Geometry check sheet. Reference: drawing and pictorial views, mm from the part's lowest x, y, z. A direction names the side the tool comes from. Round coordinates to 2 decimals unless told otherwise and drop trailing zeros. Loops run counter-clockwise (first coordinate to the right, second up) from the corner with the lowest first, then second, coordinate; pieces in that order, holes last. Notation, with made-up numbers: (-12.75, 76) -> (11.25, 76) arc R20 cw to (11.25, 87) -> close; hole circle Ø5 at (-23, -10.75). An arc over 180 degrees is marked (long way). Use one line per item in the form item = value. Start each with the question number.
(1) Material ranges on probe 1 along Z at (x, y) = (5.5, 6.5); probe 2 along Y at (x, z) = (3, 18.75); probe 3 along Y at (x, z) = (17, 18.75), recorded low to high. Write a range as [from, to].
(2) Draft check along X on the marked faces 1, 2 and 3. Enter one of: released by +X, released by -X, zero draft, split by the parting line, or undercut.
(3) Sectioned sample at B-B (x = 3). Record the cut outline in (y, z).
(4) Sectioned sample at D-D (x = 10). Record the cut outline in (y, z), and give its area (3 significant figures).
(5) Sectioned sample at C-C (z = 15.5). Record the cut outline in (x, y), and give its area (3 significant figures).
(6) Set-up check for the marked faces 4, 5 and 6: record each of +Z, -Z, +X, -X, +Y, -Y from which the full face is reachable in a straight line by a thin tool's end or side.
(7) Go/stop test with flat-tipped pins: pin 1 (1 mm diameter, centred on x = 10.5, z = 11, fed in from -Y); pin 2 (5 mm diameter, centred on y = 21, z = 6, fed in from +X) (3 decimals); pin 3 (1 mm diameter, centred on x = 9.5, y = 15, fed in from +Z). Record where each tip stops, or that it passes through.
(8) Sectioned sample at A-A (z = 24.25). Record the cut outline in (x, y).
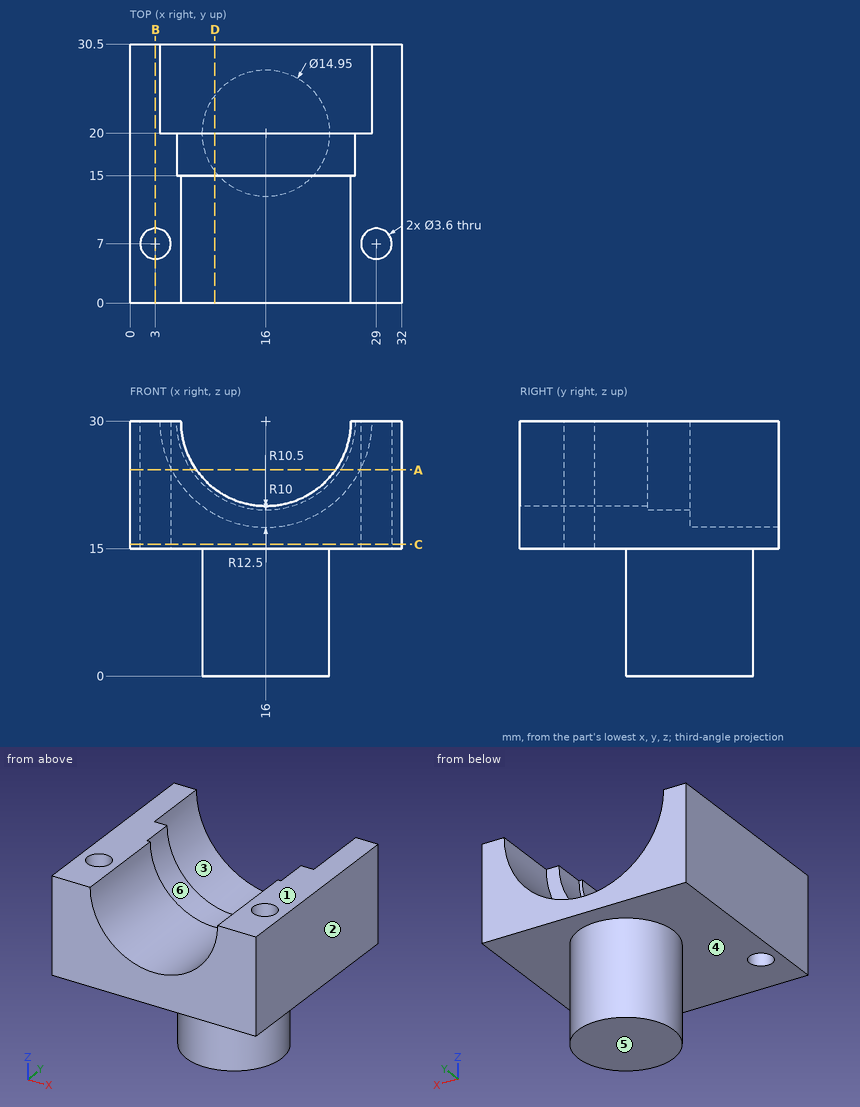
Checks:
q1.probe_1 = [15, 30]
q1.probe_2 = [0, 5.2], [8.8, 30.5]
q1.probe_3 = [0, 20]
q2.face_1 = zero draft
q2.face_2 = released by +X
q2.face_3 = undercut
q3.outline = (0, 15) -> (5.2, 15) -> (5.2, 30) -> (0, 30) -> close; (8.8, 15) -> (30.5, 15) -> (30.5, 30) -> (8.8, 30) -> close
q4.outline = (0, 15) -> (15.54, 15) -> (15.54, 0) -> (24.46, 0) -> (24.46, 15) -> (30.5, 15) -> (30.5, 19.03) -> (20, 19.03) -> (20, 21.38) -> (15, 21.38) -> (15, 22) -> (0, 22) -> close
q4.area = 313 mm2
q5.outline = (0, 0) -> (32, 0) -> (32, 30.5) -> (0, 30.5) -> close; hole circle Ø3.6 at (3, 7); hole circle Ø3.6 at (29, 7)
q5.area = 956 mm2
q6.face_4 = -Z
q6.face_5 = -Z, +X, -X, +Y, -Y
q6.face_6 = +Z, +Y
q7.pin_1 = 14.44
q7.pin_2 = 23.475
q7.pin_3 = 22.86
q8.outline = (0, 0) -> (7.82, 0) -> (7.82, 15) -> (7.21, 15) -> (7.21, 20) -> (4.9, 20) -> (4.9, 30.5) -> (0, 30.5) -> close; (24.18, 0) -> (32, 0) -> (32, 30.5) -> (27.1, 30.5) -> (27.1, 20) -> (24.79, 20) -> (24.79, 15) -> (24.18, 15) -> close; hole circle Ø3.6 at (3, 7); hole circle Ø3.6 at (29, 7)
